from build123d import *

# Parameters (mm, degrees)
EXTRUDE_1_DEPTH     = 20
CUT_EXTRUDE_1_DEPTH = 2
EXTRUDE_START       = 2
EXTRUDE_2_DEPTH     = 2
EXTRUDE_3_DEPTH     = 33
CUT_EXTRUDE_4_DEPTH = 22.5
EXTRUDE_5_DEPTH     = 20
SKETCH_11_R         = 8
EXTRUDE_6_DEPTH     = 6
SKETCH_13_W         = 5
SKETCH_13_H         = 22.035528512
CUT_EXTRUDE_5_DEPTH = 40
SKETCH_14_R         = 2.5
CUT_EXTRUDE_6_DEPTH = 20


with BuildPart() as part:
    # 草图1 → 凸台-拉伸1 (new, symmetric)
    with BuildSketch(Plane.XY):
        with BuildLine():
            Line((14.229470778, 51.299168583), (-6.23969278, 34.123500992))
            ThreePointArc((-6.23969278, 34.123500992), (-8.472070721, 31.463056561), (-9.659894213, 28.199538337))
            Line((-9.659894213, 28.199538337), (-22.919720748, -47.000674818))
            Line((-22.919720748, -47.000674818), (-20.950105242, -47.347971173))
            Line((-20.950105242, -47.347971173), (-7.816684243, 27.135360565))
            ThreePointArc((-7.816684243, 27.135360565), (-6.628860751, 30.398878788), (-4.39648281, 33.059323219))
            Line((-4.39648281, 33.059323219), (14.957411246, 49.299168583))
            Line((14.957411246, 49.299168583), (14.229470778, 51.299168583))
        make_face()
    extrude(amount=EXTRUDE_1_DEPTH, both=True)

    # 草图3 → 切除-拉伸1 (cut)
    with BuildSketch(Plane(origin=(-14.191017833, 2.502259328, 0), x_dir=(0, 0, 1), z_dir=(-0.9848077530122074, 0.17364817766693458, 0))):
        Polygon((13, -50.266596698), (20, -50.266596698), (20, 8.093700959), align=None)
    cut_extrude_1 = extrude(amount=-CUT_EXTRUDE_1_DEPTH, mode=Mode.SUBTRACT)

    # 镜向1: 切除-拉伸1 across plane
    add(cut_extrude_1.mirror(Plane.XY), mode=Mode.SUBTRACT)

    # 草图4 → 凸台-拉伸2 (add)
    with BuildSketch(Plane.XY.offset(20).offset(EXTRUDE_START)):
        with BuildLine():
            Line((-12.785561411, 10.472998783), (17.743478932, 5.089905275))
            Line((17.743478932, 5.089905275), (26.15106548, 18.544856334))
            Line((26.15106548, 18.544856334), (14.229470778, 51.299168583))
            Line((14.229470778, 51.299168583), (-6.23969278, 34.123500992))
            ThreePointArc((-6.23969278, 34.123500992), (-8.472070721, 31.463056561), (-9.659894213, 28.199538337))
            Line((-9.659894213, 28.199538337), (-12.785561411, 10.472998783))
        make_face()
    extrude_2 = extrude(amount=-EXTRUDE_2_DEPTH)

    # 草图5 → 凸台-拉伸3 (add)
    with BuildSketch(Plane(origin=(-14.191017833, 2.502259328, 0), x_dir=(0, 0, 1), z_dir=(-0.9848077530122074, 0.17364817766693458, 0))):
        Polygon((22, 8.093700959), (15, -50.266596698), (13, -50.266596698), (20, 8.093700959), align=None)
    extrude_3 = extrude(amount=-EXTRUDE_3_DEPTH)

    # 镜向3: 凸台-拉伸2, 凸台-拉伸3 across plane
    add(extrude_2.mirror(Plane.XY))
    add(extrude_3.mirror(Plane.XY))

    # 草图8 → 切除-拉伸4 (cut, symmetric)
    with BuildSketch(Plane.XY):
        with BuildLine():
            Line((17.743478932, 5.089905275), (5.494596432, -9.126276461))
            ThreePointArc((5.494596432, -9.126276461), (4.035122352, -11.368395051), (3.222317206, -13.917219909))
            Line((3.222317206, -13.917219909), (-3.223565687, -50.473638371))
            Line((-3.223565687, -50.473638371), (21.878971758, -54.899893007))
            Line((21.878971758, -54.899893007), (32.013131095, 2.573780594))
            Line((32.013131095, 2.573780594), (17.743478932, 5.089905275))
        make_face()
    extrude(amount=CUT_EXTRUDE_4_DEPTH, both=True, mode=Mode.SUBTRACT)

    # 草图10 → 凸台-拉伸5 (add)
    with BuildSketch(Plane(origin=(-14.191017833, 2.502259328, 0), x_dir=(0, 0, 1), z_dir=(-0.9848077530122074, 0.17364817766693458, 0))):
        Polygon((-15, -50.266596698), (15, -50.266596698), (14.760110888, -52.266596698), (-14.760110888, -52.266596698), align=None)
    extrude(amount=-EXTRUDE_5_DEPTH)

    # 草图11 → 凸台-拉伸6 (add)
    with BuildSketch(Plane(origin=(-9.075999269, -51.472549652, 0), x_dir=(0.9848077530122074, -0.17364817766693455, 0), z_dir=(-0.17364817766693455, -0.9848077530122074, 0))):
        with Locations(Location((-4.409937158, 0, 0), (0, 0, 180))):
            Circle(SKETCH_11_R)
    extrude(amount=EXTRUDE_6_DEPTH)

    # 草图12 → 旋转1 (revolve)
    with BuildSketch(Plane.XY, mode=Mode.PRIVATE) as revolve_1_sk:
        with BuildLine():
            Line((-14.460828639, -56.615618619), (-6.582366615, -58.00480404))
            ThreePointArc((-6.582366615, -58.00480404), (-9.872217148, -63.168834973), (-15.85001406, -64.494080643))
            Line((-15.85001406, -64.494080643), (-14.460828639, -56.615618619))
        make_face()
    revolve(revolve_1_sk.sketch.rotate(Axis((-14.460828639, -56.615618619, 0), (-0.17364817766693416, -0.9848077530122075, 0)), 180), axis=Axis((-14.460828639, -56.615618619, 0), (-0.17364817766693416, -0.9848077530122075, 0)))

    # 草图13 → 切除-拉伸5 (cut)
    with BuildSketch(Plane(origin=(-14.191017833, 2.502259328, 0), x_dir=(0, 0, 1), z_dir=(-0.9848077530122074, 0.17364817766693458, 0))):
        with Locations((0, -63.284360954)):
            Rectangle(SKETCH_13_W, SKETCH_13_H)
    extrude(amount=-CUT_EXTRUDE_5_DEPTH, mode=Mode.SUBTRACT)

    # 草图14 → 切除-拉伸6 (cut, symmetric)
    with BuildSketch(Plane.XY):
        with Locations(Location((-14.460828639, -56.615618619, 0), (0, 0, 350))):
            Circle(SKETCH_14_R)
    extrude(amount=CUT_EXTRUDE_6_DEPTH, both=True, mode=Mode.SUBTRACT)


solid = part.part
Work out the finished part from the listing and answer in its coordinate system (mm). A direction names the side the tool comes from. Round coordinates to 2 decimals unless told otherwise and drop trailing zeros. Order: outer loops, then holes, each group sorted by start corner. A loop starts at its lowest first (then second) coordinate and runs counter-clockwise, first axis right, second up. Notation, with made-up numbers: M -24,35.5 L 4,35.5 A19 ccw 4,58.5 Z; hole C 47,11 d10. An arc over 180 degrees is marked long. Put each result on its own line as item: value. Start each with the question number.
Q1. Flat-ended cylindrical pins translate along their axes: pin 1 (10 mm diameter, centred on x = -16.5, y = -31.5, fed in from -Z); pin 2 (6 mm diameter, centred on x = -14.46, y = -56.62, fed in from +Z); pin 3 (10 mm diameter, centred on y = 8, z = 2, fed in from -X); pin 4 (4.5 mm diameter, centred on x = -14.46, y = -56.62, fed in from +Z). Find the tip coordinate at first contact, or state that the pin passes through.
Q2. Section A-A, the plane z = -10.5 is taken. Write down the section's boundary in (x, y), and give its area (3 significant figures).
Q3. A tool of negligible diameter and unlimited length cuts with its end or side. For faces 4 (the flat face through (4.1, 42.8, -0.3)), 5 (the flat face through (7, 23, -20)), 6 (the flat face through (-13, -59, 2.5)), from which of +Z, -Z, +X, -X, +Y, -Y can it reach the whole face along a straight path? Write none if from no direction.
Q4. For a pull along X with two mould halves and no side action, classify faces 1 (the flat face through (6, 23, 22)), 2 (the cylindrical face through (-14.35, -54.12, -5.22)), 3 (the flat face through (-14.475, -10.628, 0.28)) as pulls with the +X half, pulls with the -X half, needs draft (parallel to the pull), parting line crosses it, or undercut.
Q5. Section D-D, the plane z = -5 is taken. Write down the section's boundary in (x, y) (1 decimal), and give its area (3 significant figures).
Q6. Straight lines are drawn through the part: L1, parallel to Z at x = 4.5, y = 11; L2, parallel to Z at x = -7.5, y = -54; L3, parallel to X at y = -16.5, z = -18.5. For each, find the intervals that lie inside material, in ascending order. Write a range as [from, to].
Q7. Section C-C, the plane y = -43.5 is taken. Write down the section's boundary in (x, z), and give its area (3 significant figures).
Q8. Section B-B, the plane x = 9.5 is taken. Write down the section's boundary in (y, z).
Findings below:
1. pin 1: stops at z = -17.56
1. pin 2: stops at z = 8
1. pin 3: stops at x = -14.1
1. pin 4: passes through
2. outline: M -23.27,-48.97 L -3.57,-52.44 L -3.22,-50.47 L -20.95,-47.35 L -7.82,27.14 A10 cw -4.4,33.06 L 14.96,49.3 L 14.23,51.3 L -6.24,34.12 A10 ccw -9.66,28.2 Z
2. area: 259 mm^2
3. face 4: +Z, -Z, -X, +Y
3. face 5: +X
3. face 6: -X, -Y
4. face 1: needs draft
4. face 2: undercut
4. face 3: pulls with the +X half
5. outline: M -23.3,-49 L -19.6,-49.6 L -20.6,-55.5 A6.2 ccw -8.3,-57.7 L -7.3,-51.8 L -3.6,-52.4 L -3.2,-50.5 L -21,-47.3 L -7.8,27.1 A10 cw -4.4,33.1 L 15,49.3 L 14.2,51.3 L -6.2,34.1 A10 ccw -9.7,28.2 Z; hole C -14.5,-56.6 d5
5. area: 375 mm^2
6. L1: z = [-22, -20], [20, 22]
6. L2: z = [-4.8, -2.5], [2.5, 4.8]
6. L3: x = [-17.54, 2.77]
7. outline: M -22.3,-15.43 L -1.99,-15.85 L -1.99,-13.85 L -20.27,-13.47 L -20.27,13.47 L -1.99,13.85 L -1.99,15.85 L -22.3,15.43 Z
7. area: 136 mm^2
8. outline: M -4.48,-20.7 L 6.54,-22 L 47.33,-22 L 47.33,22 L 6.54,22 L -4.48,20.7 L -4.48,18.7 L 6.54,20 L 44.72,20 L 44.72,-20 L 6.54,-20 L -4.48,-18.7 Z
